Input: dimensioned drawing with shaded views. Units: mm. Origin: part minimum x, y, z. A direction names the side the tool comes from. Round coordinates to 2 decimals unless told otherwise and drop trailing zeros. Loops run counter-clockwise (first coordinate to the right, second up) from the corner with the lowest first, then second, coordinate; pieces in that order, holes last. Notation, with made-up numbers: M 48,-26.5 L 107,-26.5 A25 ccw 107,-10.5 Z; hole C 84.5,-17 d3. An arc over 180 degrees is marked long. Use one line per item in the form item = value. Start each with the question number.
Q1. Access query for the marked faces 1, 2, 3 and 4. Directions: +Z, -Z, +X, -X, +Y, -Y. A direction counts if a zero-diameter tool reaches every point of the face in a straight line with its end or side. Return the directions, or none.
Q2. First-contact query: P1, Ø2, axis at x = 6.5, z = 7.5, coming from the -Y side; P2, Ø2, axis at x = 8.5, y = 18.5, coming from the -Z side (3 decimals); P3, Ø3, axis at x = 11, y = 12.5, coming from the -Z side. Flat tips, straight axial feed; report the tip coordinate or a pass-through.
Q3. Section query B-B, the plane z = 7. Output: boundary loops of the cut face in (x, y), and give its area (3 significant figures).
Q4. Mould query, pull axis X, two halves, no side actions, for the marked faces 5, 6 and 7. Classes: pulls with the +X half, pulls with the -X half, needs draft (parallel to the pull), parting line crosses it, or undercut.
Q5. Section query D-D, the plane x = 16. Output: boundary loops of the cut face in (y, z), and give its area (3 significant figures).
Q6. Section query A-A, the plane x = 12. Output: boundary loops of the cut face in (y, z), and give its area (4 significant figures).
Q7. Ray query, line 1 along X through (y, z) = (4.75, 6.5); line 2 along Y through (x, z) = (15.25, 8); line 3 along Y through (x, z) = (14.5, 6.5). Return the intervals inside material, ascending.
Q8. Section query C-C, the plane y = 16. Output: boundary loops of the cut face in (x, z).
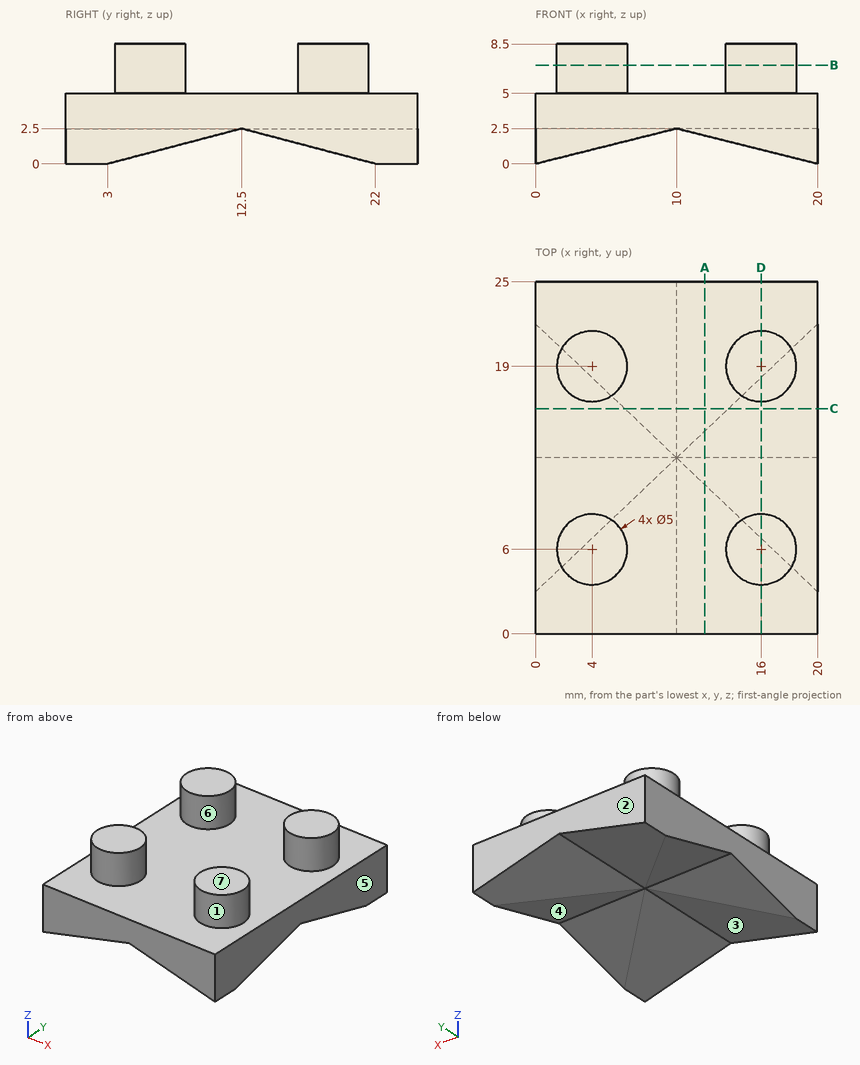
Results found:
q1.face_1 = +Z
q1.face_2 = +Z, -Z, +X, -X, +Y
q1.face_3 = -Z, +Y, -Y
q1.face_4 = -Z, +X, -X
q2.P1 = 4
q2.P2 = 1.875
q2.P3 = 2.13
q3.outline = C 4,6 d5; C 4,19 d5; C 16,6 d5; C 16,19 d5
q3.area = 78.5 mm²
q4.face_5 = pulls with the +X half
q4.face_6 = undercut
q4.face_7 = needs draft
q5.outline = M 0,1 L 6.8,1 L 12.5,2.5 L 18.2,1 L 25,1 L 25,5 L 21.5,5 L 21.5,8.5 L 16.5,8.5 L 16.5,5 L 8.5,5 L 8.5,8.5 L 3.5,8.5 L 3.5,5 L 0,5 Z
q5.area = 126 mm²
q6.outline = M 0,2 L 10.6,2 L 12.5,2.5 L 14.4,2 L 25,2 L 25,5 L 0,5 Z
q6.area = 74.05 mm²
q7.line_1 = 1.83 to 6.17, 13.83 to 18.17
q7.line_2 = 3.62 to 8.38, 16.62 to 21.38
q7.line_3 = 4 to 8, 17 to 21
q8.outline = M 0,1.58 L 6.32,1.58 L 10,2.5 L 13.68,1.58 L 20,1.58 L 20,5 L 0,5 Z
